from build123d import *

# Parameters (mm, degrees)
SKETCH1_W                 = 267.22
SKETCH1_H                 = 361.68
SKETCH1_R                 = 3.57
BOSS_EXTRUDE1_DEPTH       = 10
SKETCH2_W                 = 101.6
SKETCH2_H                 = 101.6
CUT_EXTRUDE1_DEPTH        = 226.066074076
LPATTERN1_COUNT           = 2
LPATTERN1_PITCH           = 110.265
LPATTERN2_COUNT           = 2
LPATTERN2_PITCH           = 110.265
LPATTERN3_COUNT           = 2
LPATTERN3_PITCH           = 114.82
LPATTERN3_COPY_1_SKETCH_W = 101.6
LPATTERN3_COPY_1_SKETCH_H = 101.6
LPATTERN3_COPY_1_DEPTH    = 226.066074076
LPATTERN3_COPY_2_SKETCH_W = 101.6
LPATTERN3_COPY_2_SKETCH_H = 101.6
LPATTERN3_COPY_2_DEPTH    = 226.066074076


with BuildPart() as part:
    # Sketch1 → Boss-Extrude1 (new body)
    with BuildSketch(Plane(origin=(0, 0, 0), x_dir=(1, 0, 0), z_dir=(0, 1, 0))):
        Rectangle(SKETCH1_W, SKETCH1_H)
        with Locations(Location((-120.91, -169.7275, 0), (0, 0, 270))):
            Circle(SKETCH1_R, mode=Mode.SUBTRACT)
        with Locations(Location((-120.91, 169.7275, 0), (0, 0, 270))):
            Circle(SKETCH1_R, mode=Mode.SUBTRACT)
        with Locations(Location((95.51, 169.7275, 0), (0, 0, 270))):
            Circle(SKETCH1_R, mode=Mode.SUBTRACT)
        with Locations(Location((95.51, -169.7275, 0), (0, 0, 270))):
            Circle(SKETCH1_R, mode=Mode.SUBTRACT)
    extrude(amount=BOSS_EXTRUDE1_DEPTH)

    # Sketch2 → Cut-Extrude1 (cut, through all)
    with BuildSketch(Plane(origin=(0, 10, 0), x_dir=(1, 0, 0), z_dir=(0, 1, 0))):
        with Locations((-70.11, 0)):
            Rectangle(SKETCH2_W, SKETCH2_H)
    cut_extrude1 = extrude(amount=-CUT_EXTRUDE1_DEPTH, mode=Mode.SUBTRACT)

    # LPattern1: Cut-Extrude1 ×2
    with Locations(*[(0, 0, -i * LPATTERN1_PITCH) for i in range(1, LPATTERN1_COUNT)]):
        add(cut_extrude1, mode=Mode.SUBTRACT)

    # LPattern2: Cut-Extrude1 ×2
    with Locations(*[(0, 0, i * LPATTERN2_PITCH) for i in range(1, LPATTERN2_COUNT)]):
        add(cut_extrude1, mode=Mode.SUBTRACT)

    # LPattern3: Cut-Extrude1 ×2
    with Locations(*[(i * LPATTERN3_PITCH, 0, 0) for i in range(1, LPATTERN3_COUNT)]):
        add(cut_extrude1, mode=Mode.SUBTRACT)

    # LPattern3 copy 1 sketch → LPattern3 copy 1 (cut, through all)
    with BuildSketch(Plane(origin=(114.82, 10, -110.265), x_dir=(1, 0, 0), z_dir=(0, 1, 0))):
        with Locations((-70.11, 0)):
            Rectangle(LPATTERN3_COPY_1_SKETCH_W, LPATTERN3_COPY_1_SKETCH_H)
    extrude(amount=-LPATTERN3_COPY_1_DEPTH, mode=Mode.SUBTRACT)

    # LPattern3 copy 2 sketch → LPattern3 copy 2 (cut, through all)
    with BuildSketch(Plane(origin=(114.82, 10, 110.265), x_dir=(1, 0, 0), z_dir=(0, 1, 0))):
        with Locations((-70.11, 0)):
            Rectangle(LPATTERN3_COPY_2_SKETCH_W, LPATTERN3_COPY_2_SKETCH_H)
    extrude(amount=-LPATTERN3_COPY_2_DEPTH, mode=Mode.SUBTRACT)


solid = part.part
Here's how the part is built. I have some questions about the finished solid (model axes, mm). Round coordinates to 2 decimals unless told otherwise and drop trailing zeros. Order: outer loops, then holes, each group sorted by start corner. A loop starts at its lowest first (then second) coordinate and runs counter-clockwise, first axis right, second up. Notation, with made-up numbers: M 25.25,-11.5 L 56.25,-11.5 A28 ccw 56.25,21.5 Z; hole C -33,25.25 d10. An arc over 180 degrees is marked long. Return JSON: item names as keys, results as strings. Group by question number.
1. If we section it at B-B on y = 5.5: State how many separate pieces and enclosed holes the cut face has, then the cut area to 3 significant figures.
2. If we mould it in two halves opening along X, with no side actions, what happens to faces 1 (the face through (-6.09, 5, 111)), 2 (the face through (95.51, 5, 1)), 3 (the face through (39, 10, -54))? For each: pulls with the +X half, pulls with the -X half, needs draft (parallel to the pull), parting line crosses it, or undercut.
3. If we section it at C-C on z = -100: List the corners of the cut face in (x, y) for me, then the cut area to 3 significant figures.
4. Please list where these lines run through material, in increasing order: probe 1 along Z at (x, y) = (-94, 7) (3 decimals); probe 2 along X at (y, z) = (7, 16).
5. I'm going to push a flat-ended pin straight in: pin 1 Ø8 at (x, z) = (105.5, -109.5) entering from -Y. Where does the tip first touch, or does it pass through?
6. If we section it at A-A on x = -57: List the corners of the cut face in (y, z) for me (3 decimals).
Reply:
{
 "1": {"separate pieces": "1", "enclosed holes": "10", "area": "34,600 mm^2"},
 "2": {"face 1": "undercut", "face 2": "undercut", "face 3": "needs draft"},
 "3": {"outline": "M -133.61,0 L -120.91,0 L -120.91,10 L -133.61,10 Z; M -19.31,0 L -6.09,0 L -6.09,10 L -19.31,10 Z; M 95.51,0 L 133.61,0 L 133.61,10 L 95.51,10 Z", "area": "640 mm^2"},
 "4": {"probe 1": "-180.84 to -161.065, -59.465 to -50.8, 50.8 to 59.465, 161.065 to 180.84", "probe 2": "-133.61 to -120.91, -19.31 to -6.09, 95.51 to 133.61"},
 "5": {"pin 1": "y = 0"},
 "6": {"outline": "M 0,-180.84 L 10,-180.84 L 10,-161.065 L 0,-161.065 Z; M 0,-59.465 L 10,-59.465 L 10,-50.8 L 0,-50.8 Z; M 0,50.8 L 10,50.8 L 10,59.465 L 0,59.465 Z; M 0,161.065 L 10,161.065 L 10,180.84 L 0,180.84 Z"}
}
